from build123d import *

# Parameters (mm, degrees)
SKETCH1_W           = 150
SKETCH1_H           = 35
BOSS_EXTRUDE1_DEPTH = 2
SKETCH2_R           = 2
FIX_HOLE_DEPTH      = 78.040573726


with BuildPart() as part:
    # Sketch1 → Boss-Extrude1 (new body)
    with BuildSketch(Plane.XY):
        Rectangle(SKETCH1_W, SKETCH1_H)
    extrude(amount=BOSS_EXTRUDE1_DEPTH)

    # Sketch2 → fix hole (cut, through all)
    with BuildSketch(Plane(origin=(0, 0, 0), x_dir=(-1, 0, 0), z_dir=(0, 0, -1))):
        with Locations(Location((30, 7.5, 0), (0, 0, 180))):
            Circle(SKETCH2_R)
        with Locations((0, 7.5)):
            Circle(SKETCH2_R)
        with Locations((-30, 7.5)):
            Circle(SKETCH2_R)
    extrude(amount=-FIX_HOLE_DEPTH, mode=Mode.SUBTRACT)


solid = part.part
Check sheet for the modelled part. Datum: model origin and axes. Units: mm. Round coordinates to 2 decimals unless told otherwise and drop trailing zeros. Loops run counter-clockwise (first coordinate to the right, second up) from the corner with the lowest first, then second, coordinate; pieces in that order, holes last. Notation, with made-up numbers: M 14.5,-36.75 L 20.5,-36.75 A13 cw 20.5,-12.75 Z; hole C 41,-25.5 d9. An arc over 180 degrees is marked long. One line per question, with ' | ' between items. Start each with the question number.
Item 1: Section check B-B (x = 0). Record the boundary of the cut face in (y, z), and give its area (3 significant figures).
Item 2: Release check for a two-part mould opening along Y. For faces 1 (the face through (-1, 0, 2)), 2 (the face through (0.26, 9.483, 0.986)) record: released by +Y, released by -Y, zero draft, split by the parting line, or undercut.
Item 3: Section check A-A (y = 7.5). Record the boundary of the cut face in (x, z).
Item 4: Scan lines: probe 1 along Y at (x, z) = (-30, 1.05); probe 2 along Y at (x, z) = (-0.5, 1.75). Record each from-to range of solid material in increasing order.
Item 5: Gauge pin test, flat end, axial feed: pin 1 Ø3 at (x, y) = (30, 7.5) entering from +Z. Record the tip position at first contact, or that the pin passes through.
Worked out:
1) outline: M -17.5,0 L 5.5,0 L 5.5,2 L -17.5,2 Z; M 9.5,0 L 17.5,0 L 17.5,2 L 9.5,2 Z | area: 62.0 mm^2
2) face 1: zero draft | face 2: undercut
3) outline: M -75,0 L -32,0 L -32,2 L -75,2 Z; M -28,0 L -2,0 L -2,2 L -28,2 Z; M 2,0 L 28,0 L 28,2 L 2,2 Z; M 32,0 L 75,0 L 75,2 L 32,2 Z
4) probe 1: -17.5 to 5.5, 9.5 to 17.5 | probe 2: -17.5 to 5.56, 9.44 to 17.5
5) pin 1: through
